Geometry check sheet. Reference: the model listing, model coordinates, mm. Round coordinates to 2 decimals unless told otherwise and drop trailing zeros. Order: outer loops, then holes, each group sorted by start corner. A loop starts at its lowest first (then second) coordinate and runs counter-clockwise, first axis right, second up.
```python
from build123d import *

# Parameters (mm, degrees)
F0_R     = 12.7
F1_DEPTH = 50.8


with BuildPart() as f1:
    # F0 (on Front) → F1 (new body)
    with BuildSketch(Plane.XZ):
        with BuildLine():
            ThreePointArc((260.35, 25.4), (267.789488, 7.439488), (285.75, 0))
            Line((285.75, 0), (406.4, 0))
            ThreePointArc((406.4, 0), (424.360512, 7.439488), (431.8, 25.4))
            Line((431.8, 25.4), (431.8, 50.8))
            ThreePointArc((431.8, 50.8), (461.557951, 122.642049), (533.4, 152.4))
            Line((533.4, 152.4), (685.8, 152.4))
            ThreePointArc((685.8, 152.4), (703.760512, 159.839488), (711.2, 177.8))
            Line((711.2, 177.8), (711.2, 400.05))
            ThreePointArc((711.2, 400.05), (703.760512, 418.010512), (685.8, 425.45))
            Line((685.8, 425.45), (6.35, 425.45))
            ThreePointArc((6.35, 425.45), (-11.610512, 418.010512), (-19.05, 400.05))
            Line((-19.05, 400.05), (-19.05, 177.8))
            ThreePointArc((-19.05, 177.8), (-11.610512, 159.839488), (6.35, 152.4))
            Line((6.35, 152.4), (158.75, 152.4))
            ThreePointArc((158.75, 152.4), (230.592049, 122.642049), (260.35, 50.8))
            Line((260.35, 50.8), (260.35, 25.4))
        make_face()
        with Locations((63.692227, 227.595572)):
            Circle(F0_R, mode=Mode.SUBTRACT)
        with Locations((114.492227, 227.595572)):
            Circle(F0_R, mode=Mode.SUBTRACT)
        with Locations((63.692227, 291.095572)):
            Circle(F0_R, mode=Mode.SUBTRACT)
        with Locations((114.492227, 291.095572)):
            Circle(F0_R, mode=Mode.SUBTRACT)
        with Locations((165.292227, 227.595572)):
            Circle(F0_R, mode=Mode.SUBTRACT)
        with Locations((216.092227, 227.595572)):
            Circle(F0_R, mode=Mode.SUBTRACT)
        with Locations((165.292227, 291.095572)):
            Circle(F0_R, mode=Mode.SUBTRACT)
        with Locations((216.092227, 291.095572)):
            Circle(F0_R, mode=Mode.SUBTRACT)
        with Locations((63.692227, 354.595572)):
            Circle(F0_R, mode=Mode.SUBTRACT)
        with Locations((114.492227, 354.595572)):
            Circle(F0_R, mode=Mode.SUBTRACT)
        with Locations((165.292227, 354.595572)):
            Circle(F0_R, mode=Mode.SUBTRACT)
        with Locations((216.092227, 354.595572)):
            Circle(F0_R, mode=Mode.SUBTRACT)
    extrude(amount=-F1_DEPTH)


solid = f1.part
```
(1) Draft check along X on faces 1 (the flat face through (609, 25, 152.4)), 2 (the cylindrical face through (171.153, 25.044, 279.828)), 3 (the flat face through (260.35, 25, 38)), 4 (the cylindrical face through (111.739, 25.044, 278.698)). Enter one of: released by +X, released by -X, zero draft, split by the parting line, or undercut.
Returned:
face 1: zero draft
face 2: undercut
face 3: released by -X
face 4: undercut
(2) Sectioned sample at C-C, the plane z = 43.5. Record the cut outline in (x, y), and give its area (3 significant figures).
Returned:
outline: (260.35, 0) - (431.8, 0) - (431.8, 50.8) - (260.35, 50.8) - close
area: 8,710 mm2
(3) Sectioned sample at D-D, the plane x = 210.5. Record the cut outline in (y, z), and give its area (3 significant figures).
Returned:
outline: (0, 138.23) - (50.8, 138.23) - (50.8, 216.19) - (0, 216.19) - close; (0, 239) - (50.8, 239) - (50.8, 279.69) - (0, 279.69) - close; (0, 302.5) - (50.8, 302.5) - (50.8, 343.19) - (0, 343.19) - close; (0, 366) - (50.8, 366) - (50.8, 425.45) - (0, 425.45) - close
area: 11,100 mm2
(4) Depth check by flat-ended pin: P1, Ø12.5, axis at y = 24, z = 34.5, coming from the -X side. Enter the tip coordinate at first touch or a pass-through.
Returned:
P1: stops at x = 260.35
(5) Sectioned sample at B-B, the plane y = 13.5. Give the number of separate pieces and of enclosed holes in the cut face, and give its area (3 significant figures).
Returned:
separate pieces: 1
enclosed holes: 12
area: 223,000 mm2
(6) Material ranges on line 1 (X direction, y = 6, z = 291.5); line 2 (X direction, y = 9, z = 346.5); line 3 (X direction, y = 20.5, z = 175), recorded low to high.
Returned:
line 1: x = -19.05 to 51, 76.39 to 101.8, 127.19 to 152.6, 177.99 to 203.4, 228.79 to 711.2
line 2: x = -19.05 to 53.91, 73.48 to 104.71, 124.28 to 155.51, 175.08 to 206.31, 225.88 to 711.2
line 3: x = -18.9 to 711.05
(7) Sectioned sample at A-A, the plane x = 120. Record the cut outline in (y, z), and give its area (3 significant figures).
Returned:
outline: (0, 152.4) - (50.8, 152.4) - (50.8, 216.15) - (0, 216.15) - close; (0, 239.04) - (50.8, 239.04) - (50.8, 279.65) - (0, 279.65) - close; (0, 302.54) - (50.8, 302.54) - (50.8, 343.15) - (0, 343.15) - close; (0, 366.04) - (50.8, 366.04) - (50.8, 425.45) - (0, 425.45) - close
area: 10,400 mm2
